Check sheet for the modelled part. Datum: model origin and axes. Units: mm. Face numbers are marked on the shaded views. A direction names the side the tool comes from. Round coordinates to 2 decimals unless told otherwise and drop trailing zeros. Write each loop counter-clockwise with the first axis right and the second up, starting at its lowest first coordinate (ties: lowest second). Pieces come first, ordered by that corner, then holes. Notation, with made-up numbers: (64, 40) -> (96, 40) arc R9 cw to (96, 48) -> close; hole circle Ø9 at (-0.75, -22.75). An arc over 180 degrees is marked (long way). One line per item, written item: value.
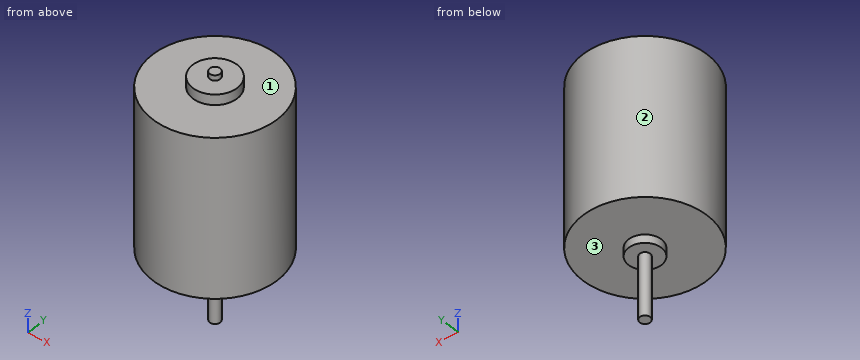
from build123d import *

# Parameters (mm, degrees)
SKETCH2_R           = 11.9
BOSS_EXTRUDE1_DEPTH = 30.5
SKETCH3_R           = 4.25
BOSS_EXTRUDE2_DEPTH = 2
SKETCH4_R           = 3.15
BOSS_EXTRUDE3_DEPTH = 1.6
SKETCH5_R           = 1
BOSS_EXTRUDE4_DEPTH = 12
BOSS_EXTRUDE5_START = 1
SKETCH6_R           = 1
BOSS_EXTRUDE5_DEPTH = 1


with BuildPart() as part:
    # Sketch2 → Boss-Extrude1 (new body)
    with BuildSketch(Plane.XY):
        with Locations(Location((0, 0, 0), (0, 0, 180))):
            Circle(SKETCH2_R)
    extrude(amount=BOSS_EXTRUDE1_DEPTH)

    # Sketch3 → Boss-Extrude2 (add)
    with BuildSketch(Plane.XY.offset(30.5)):
        Circle(SKETCH3_R)
    extrude(amount=BOSS_EXTRUDE2_DEPTH)

    # Sketch4 → Boss-Extrude3 (add)
    with BuildSketch(Plane(origin=(0, 0, 0), x_dir=(-1, 0, 0), z_dir=(0, 0, -1))):
        Circle(SKETCH4_R)
    extrude(amount=BOSS_EXTRUDE3_DEPTH)

    # Sketch5 → Boss-Extrude4 (add)
    with BuildSketch(Plane(origin=(0, 0, -1.6), x_dir=(-1, 0, 0), z_dir=(0, 0, -1))):
        Circle(SKETCH5_R)
    extrude(amount=BOSS_EXTRUDE4_DEPTH)

    # Sketch6 → Boss-Extrude5 (add)
    with BuildSketch(Plane.XY.offset(32.5).offset(BOSS_EXTRUDE5_START)):
        with Locations(Location((0, 0, 0), (0, 0, 180))):
            Circle(SKETCH6_R)
    extrude(amount=-BOSS_EXTRUDE5_DEPTH)


solid = part.part
Item 1: Sectioned sample at D-D on y = -9.5. Enter the section's corners in (x, z), and give its area (3 significant figures).
Answer:
outline: (-7.17, 0) -> (7.17, 0) -> (7.17, 30.5) -> (-7.17, 30.5) -> close
area: 437 mm^2
Item 2: Sectioned sample at A-A on x = 0. Enter the section's corners in (y, z).
Answer:
outline: (-11.9, 0) -> (-3.15, 0) -> (-3.15, -1.6) -> (-1, -1.6) -> (-1, -13.6) -> (1, -13.6) -> (1, -1.6) -> (3.15, -1.6) -> (3.15, 0) -> (11.9, 0) -> (11.9, 30.5) -> (4.25, 30.5) -> (4.25, 32.5) -> (1, 32.5) -> (1, 33.5) -> (-1, 33.5) -> (-1, 32.5) -> (-4.25, 32.5) -> (-4.25, 30.5) -> (-11.9, 30.5) -> close
Item 3: Depth check by flat-ended pin: P1, Ø5, axis at x = 5.5, y = -5.5, coming from the -Z side; P2, Ø10, axis at y = -6.5, z = 2, coming from the +X side; P3, Ø8, axis at x = 6, z = 18, coming from the -Y side. Enter the tip coordinate at first touch or a pass-through.
Answer:
P1: stops at z = 0
P2: stops at x = 11.81
P3: stops at y = -11.73
Item 4: Tool access check on the marked faces 1, 2 and 3. Record the directions out of +Z, -Z, +X, -X, +Y, -Y that give a thin tool (end or side, any length) a straight path to the whole face; none if there is none.
Answer:
face 1: +Z
face 2: +Z, -Z
face 3: -Z
Item 5: Sectioned sample at C-C on z = 22. Enter the section's corners in (x, y).
Answer:
outline: circle Ø23.8 at (0, 0)
Item 6: Thickness scan on line 1 (Z direction, x = 8.75, y = -5.5); line 2 (Y direction, x = -0.25, z = 24.5); line 3 (Z direction, x = 1.25, y = -2.5). Record the ranges inside material, lowest first.
Answer:
line 1: z = 0 to 30.5
line 2: y = -11.9 to 11.9
line 3: z = -1.6 to 32.5
